```python
from build123d import *

# Parameters (mm, degrees)
SKETCH_1_R      = 1.5
SKETCH_1_W      = 8.2
SKETCH_1_H      = 2.2
EXTRUDE_1_DEPTH = 2


with BuildPart() as part:
    # 草图1 → 凸台-拉伸1 (new body)
    with BuildSketch(Plane.XY):
        Polygon((-47.766155614, -53.199512395), (-47.766155614, -54.699512395), (-45.166155614, -54.699512395), (-45.166155614, -53.199512395), (-42.166155614, -53.199512395), (-42.166155614, -50.199512395), (-45.166155614, -50.199512395), (-45.166155614, -48.699512395), (-47.766155614, -48.699512395), (-47.766155614, -50.199512395), (-50.266155614, -50.199512395), (-50.266155614, -45.199512395), (-35.266155614, -45.199512395), (-35.266155614, -83.137012395), (30.733844386, -83.137012395), (30.733844386, -45.199512395), (45.733844386, -45.199512395), (45.733844386, -50.199512395), (43.233844386, -50.199512395), (43.233844386, -48.699512395), (40.633844386, -48.699512395), (40.633844386, -50.199512395), (37.633844386, -50.199512395), (37.633844386, -53.199512395), (40.633844386, -53.199512395), (40.633844386, -54.699512395), (43.233844386, -54.699512395), (43.233844386, -53.199512395), (45.733844386, -53.199512395), (45.733844386, -79.137012395), (48.733844386, -79.137012395), (48.733844386, -87.137012395), (45.733844386, -87.137012395), (45.733844386, -118.574512395), (-50.266155614, -118.574512395), (-50.266155614, -87.137012395), (-53.266155614, -87.137012395), (-53.266155614, -79.137012395), (-50.266155614, -79.137012395), (-50.266155614, -53.199512395), align=None)
        with Locations((-35.266155614, -114.574512395)):
            Circle(SKETCH_1_R, mode=Mode.SUBTRACT)
        with Locations(Location((30.733844386, -114.574512395, 0), (0, 0, 180))):
            Circle(SKETCH_1_R, mode=Mode.SUBTRACT)
        with Locations((-2.266155614, -100.855762395)):
            Circle(SKETCH_1_R, mode=Mode.SUBTRACT)
        with Locations((-2.266155614, -90.855762395)):
            Circle(SKETCH_1_R, mode=Mode.SUBTRACT)
        with Locations((-20.016155614, -114.574512396)):
            Rectangle(SKETCH_1_W, SKETCH_1_H, mode=Mode.SUBTRACT)
        with Locations((15.483844386, -114.574512396)):
            Rectangle(SKETCH_1_W, SKETCH_1_H, mode=Mode.SUBTRACT)
    extrude(amount=EXTRUDE_1_DEPTH)


solid = part.part
```
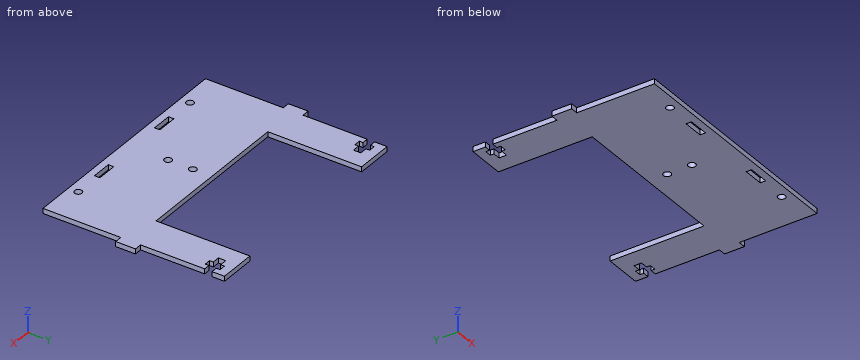
Could you check a few things on this model? Use its own coordinates, in mm. Round coordinates to 2 decimals unless told otherwise and drop trailing zeros. Write each loop counter-clockwise with the first axis right and the second up, starting at its lowest first coordinate (ties: lowest second). Pieces come first, ordered by that corner, then holes.
(1) Suppose I cut it at D-D on z = 1.3. State how many separate pieces and enclosed holes the cut face has, and give its area (3 significant figures).
Findings below:
separate pieces: 1
enclosed holes: 6
area: 4,460 mm2
(2) Suppose I cut it at A-A on y = -52. Write out the boundary of the cut face in (x, z).
Findings below:
outline: (-42.17, 0) - (-35.27, 0) - (-35.27, 2) - (-42.17, 2) - close; (30.73, 0) - (37.63, 0) - (37.63, 2) - (30.73, 2) - close
(3) If I drill on probe 1 along Y at (x, z) = (-2.5, 0.85); probe 2 along X at (y, z) = (-50, 1.1); probe 3 along Y at (x, z) = (-44.5, 0.8), over which ranges is the centre line in solid material (lowest first)?
Findings below:
probe 1: y = -118.57 to -102.34, -99.37 to -92.34, -89.37 to -83.14
probe 2: x = -50.27 to -47.77, -45.17 to -35.27, 30.73 to 40.63, 43.23 to 45.73
probe 3: y = -118.57 to -53.2, -50.2 to -45.2
(4) For pin 1 (0.6 mm diameter, centred on y = -114.5, z = 1.5, fed in from +X); pin 2 (1 mm diameter, centred on x = 46.5, z = 0.5, fed in from +Y); pin 3 (0.6 mm diameter, centred on y = -47, z = 1, fed in from -X), each with a flat end and sliding along its axis, tell me the tip position at first contact or that it passes through.
Findings below:
pin 1: stops at x = 45.73
pin 2: stops at y = -79.14
pin 3: stops at x = -50.27
(5) Suppose I cut it at C-C on y = -96.5. Write out the boundary of the cut face in (x, z), and give its area (3 significant figures).
Findings below:
outline: (-50.27, 0) - (45.73, 0) - (45.73, 2) - (-50.27, 2) - close
area: 192 mm2
(6) Suppose I cut it at B-B on x = -22. Write out the boundary of the cut face in (y, z), and give its area (3 significant figures).
Findings below:
outline: (-118.57, 0) - (-115.67, 0) - (-115.67, 2) - (-118.57, 2) - close; (-113.47, 0) - (-83.14, 0) - (-83.14, 2) - (-113.47, 2) - close
area: 66.5 mm2
